The model under review builds one solid part; all positions refer to its coordinate system, in mm. Face numbers are marked on the shaded views. A direction names the side the tool comes from. Coordinates: 2 decimals unless noted, no trailing zeros. Loops run counter-clockwise (first coordinate to the right, second up) from the corner with the lowest first, then second, coordinate; pieces in that order, holes last. Notation, with made-up numbers: M 67.5,27 L 115.5,27 A19 cw 115.5,53 Z; hole C 80.5,-36 d5. An arc over 180 degrees is marked long. Return JSON: item names as keys, results as strings.
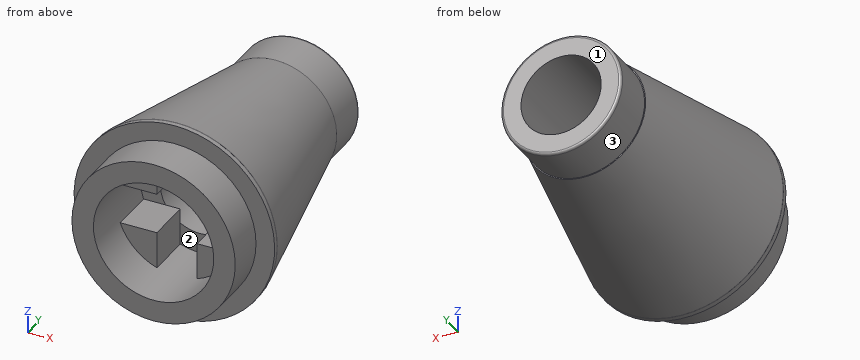
Autodesk Inventor part; units mm, degrees
ref_plane "YZ Plane" through (0, 0, 0) normal (1, 0, 0) x (0, 1, 0)
ref_plane "XZ Plane" through (0, 0, 0) normal (0, 1, 0) x (-1, 0, 0)
ref_plane "XY Plane" through (0, 0, 0) normal (0, 0, 1) x (1, 0, 0)
sketch "Sketch11" plane through (0, 0, 0) normal (1, 0, 0) x (0, 1, 0)
  line L0 (0, 3.2569) -> (1.6, 3.2569)
  line L1 (1.6, 4) -> (1.8, 4)
  line L2 (-2.24, 0) -> (13.44, 0)
  line L3 (1.6, 3.2569) -> (1.6, 4)
  line L4 (1.8, 4) -> (9.6, 2.4)
  line L5 (9.6, 2.4) -> (11.2, 2.4)
  line L6 (11.2, 2.4) -> (11.2, 1.6)
  line L7 (11.2, 1.6) -> (3.6, 1.6)
  line L8 (3.6, 1.6) -> (3.6, 2.4)
  line L9 (3.6, 2.4) -> (0, 2.4)
  line L10 (0, 2.4) -> (0, 3.2569)
  line L11 (9.6, 2.4) -> (9.4, 2.4)
  line L12 (9.4, 2.4) -> (9.4, 2.441)
  point P0 (0, 0)
  dimension "d99" = 4.8
  dimension "d100" = 1.6
  dimension "d101" = 6.5137
  dimension "d102" = 8
  dimension "d104" = 3.2
  dimension "d105" = 4.8
  dimension "d106" = 1.6
  dimension "d107" = 9.6
  dimension "d109" = 3.6
  dimension "d110" = 0.2
  dimension "d116" = 1.8
revolve "Revolution1" add sketch "Sketch11" angle 360 about axis through (0, -10, 0) along (0, 1, 0) contours L0 L3 L1 L4 L12 L11 L5 L6 L7 L8 L9 L10
fillet "Fillet1" radius 0.1 2 edges at (0, 11.2, -2.4) (0, 1.8, -4)
sketch "Sketch12" plane through (0, 3.6, 0) normal (0, -1, 0) x (1, 0, 0)
  circle A0 centre (0, 0) radius 2.4
  line L0 (-0.8, 2.2627) -> (-0.8, 0.8)
  line L1 (-0.8, 0.8) -> (-2.2627, 0.8)
  line L2 (-2.2627, -0.8) -> (-0.8, -0.8)
  line L3 (-0.8, -0.8) -> (-0.8, -2.2627)
  line L4 (0.8, -2.2627) -> (0.8, -0.8)
  line L5 (0.8, -0.8) -> (2.2627, -0.8)
  line L6 (2.2627, 0.8) -> (0.8, 0.8)
  line L7 (0.8, 0.8) -> (0.8, 2.2627)
  dimension "d111" = 1.6
extrude "Extrusion7" add sketch "Sketch12" along normal blind 1.8 contours L6 L7 A0 | A0 L4 L5 | L0 L1 A0 | A0 L2 L3
equation "\"d99\" = kd"
equation "\"d100\" = 0.333333 * lh - topthk"
equation "\"d101\" = tubeod"
equation "\"d102\" = lu"
equation "\"d104\" = rd"
equation "\"d105\" = kd"
equation "\"d106\" = knobh"
equation "\"d107\" = lh"
equation "\"d22\" = lf"
equation "\"d111\" = axlet"
properties part number "59900-Black" material "ABS Plastic"
1. Insertion check: pin 1 Ø0.8 at (x, z) = (0, -1.5) entering from -Y; pin 2 Ø4 at (y, z) = (4, -1) entering from -X; pin 3 Ø1.2 at (x, y) = (-1.5, 3) entering from +Z. Each pin has a flat end and moves straight along its axis. Give the tip position at first contact, or say it passes through.
Check values:
{"pin 1": "y = 3.6", "pin 2": "x = -3.92", "pin 3": "z = 3.69"}
2. Add section C-C on y = 6.5. Give the boundary of the cut face in (x, z), plus the area to 3 significant figures.
Check values:
{"outline": "C 0,0 d6.07; hole C 0,0 d3.2", "area": "20.9 mm²"}
3. Add section A-A on y = 2.5. Give the boundary of the cut face in (x, z), plus the area to 3 significant figures.
Check values:
{"outline": "C 0,0 d7.71; hole M -2.26,-0.8 L -0.8,-0.8 L -0.8,-2.26 A2.4 ccw 0.8,-2.26 L 0.8,-0.8 L 2.26,-0.8 A2.4 ccw 2.26,0.8 L 0.8,0.8 L 0.8,2.26 A2.4 ccw -0.8,2.26 L -0.8,0.8 L -2.26,0.8 A2.4 ccw Z", "area": "34.2 mm²"}
4. Add section B-B on y = 5. Give the boundary of the cut face in (x, z), plus the area to 3 significant figures.
Check values:
{"outline": "C 0,0 d6.69; hole C 0,0 d3.2", "area": "27.1 mm²"}
5. Machinability: for the marked faces 1, 2 and 3, which of the approach directions +Z, -Z, +X, -X, +Y, -Y give a long, thin tool a straight path to every point of the face, cutting with its end or side? Answer none if there is none.
Check values:
{"face 1": "+Z, -Z, +X, -X, +Y", "face 2": "-Y", "face 3": "+Y"}
6. To check wall thickness, follow line 1 (X direction, y = 0.8, z = 0); line 2 (Z direction, x = 0, y = 8.5); line 3 (X direction, y = 9.5, z = 0). State the ranges of each line that lie inside material, in increasing order.
Check values:
{"line 1": "-3.26 to -2.4, 2.4 to 3.26", "line 2": "-2.63 to -1.6, 1.6 to 2.63", "line 3": "-2.4 to -1.6, 1.6 to 2.4"}
